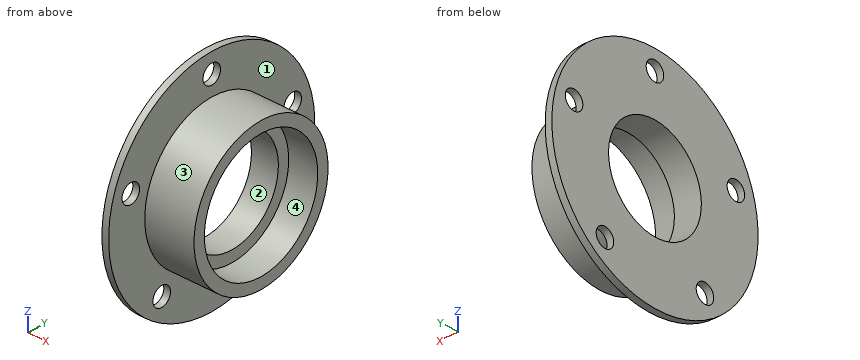
from build123d import *

# Parameters (mm, degrees)
F3_D     = 8.5
F3_DEPTH = 49.5
F3_TIP   = 2.5536576309


# Not quite as in the source:
# - a feature names something its author has since deleted; it is built from what else it names


with BuildPart() as f1:
    # F0 (on Front) → F1 (revolve)
    with BuildSketch(Plane.XZ):
        Polygon((-15.4332816247, 27.5), (-2.4332816247, 27.5), (-2.4332816247, 32.5), (-24.5, 32.5), (-24.5, 50), (-27.5, 50), (-27.5, 22.5), (-15.4332816247, 22.5), align=None)
    revolve(axis=Axis((-62.9697144032, 0, 0), (-1, 0, 0)))

    # F3
    with Locations(Plane(origin=(-27.5, 0, 0), x_dir=(0, -1, 0), z_dir=(-1, 0, 0))):
        with Locations((0, 41.25), (39.2310812972, 12.746951018), (24.2461416571, -33.371951018), (-24.2461416571, -33.371951018), (-39.2310812972, 12.746951018)):
            Hole(F3_D / 2, depth=F3_DEPTH)
            with Locations((0, 0, -(F3_DEPTH + F3_TIP / 2))):  # 118° drill point
                Cone(0, F3_D / 2, F3_TIP, mode=Mode.SUBTRACT)


solid = f1.part
Design review of the part built by this model. Coordinates are the model's own, in mm. Face numbers are marked on the shaded views. Round coordinates to 2 decimals unless told otherwise and drop trailing zeros. Loops run counter-clockwise (first coordinate to the right, second up) from the corner with the lowest first, then second, coordinate; pieces in that order, holes last. Notation, with made-up numbers: M 48,23.25 L 79,23.25 A26 ccw 79,61.25 Z; hole C 13,-25 d4. An arc over 180 degrees is marked long. Answer as a JSON object with one key per item and string values.
Item 1: We need section B-B on z = 11.5. Give the boundary of the cut face in (x, y), and give its area (3 significant figures).
Answer sheet:
{"outline": "M -27.5,-48.66 L -24.5,-48.66 L -24.5,-43.29 L -27.5,-43.29 Z; M -27.5,-35.17 L -24.5,-35.17 L -24.5,-30.4 L -2.43,-30.4 L -2.43,-24.98 L -15.43,-24.98 L -15.43,-19.34 L -27.5,-19.34 Z; M -27.5,19.34 L -15.43,19.34 L -15.43,24.98 L -2.43,24.98 L -2.43,30.4 L -24.5,30.4 L -24.5,35.17 L -27.5,35.17 Z; M -27.5,43.29 L -24.5,43.29 L -24.5,48.66 L -27.5,48.66 Z", "area": "469 mm^2"}
Item 2: We need section C-C on y = -15.5. Give the boundary of the cut face in (x, z).
Answer sheet:
{"outline": "M -27.5,-47.54 L -24.5,-47.54 L -24.5,-28.57 L -2.43,-28.57 L -2.43,-22.72 L -15.43,-22.72 L -15.43,-16.31 L -27.5,-16.31 Z; M -27.5,16.31 L -15.43,16.31 L -15.43,22.72 L -2.43,22.72 L -2.43,28.57 L -24.5,28.57 L -24.5,47.54 L -27.5,47.54 Z"}
Item 3: The part is to be moulded in two halves that separate along Z. For the marked faces 1, 2, 3 and 4, say which applies: pulls with the +Z half, pulls with the -Z half, needs draft (parallel to the pull), parting line crosses it, or undercut.
Answer sheet:
{"face 1": "needs draft", "face 2": "undercut", "face 3": "parting line crosses it", "face 4": "undercut"}
Item 4: We need section D-D on z = 0. Give the boundary of the cut face in (x, y).
Answer sheet:
{"outline": "M -27.5,-50 L -24.5,-50 L -24.5,-32.5 L -2.43,-32.5 L -2.43,-27.5 L -15.43,-27.5 L -15.43,-22.5 L -27.5,-22.5 Z; M -27.5,22.5 L -15.43,22.5 L -15.43,27.5 L -2.43,27.5 L -2.43,32.5 L -24.5,32.5 L -24.5,50 L -27.5,50 Z"}
Item 5: Clearance check with flat-ended pins moving along their axes: P1, Ø1.5, axis at x = -7, y = 29.5, coming from the +Z side; P2, Ø4, axis at x = -10.5, y = -3.5, coming from the -Z side; P3, Ø2, axis at x = -6, z = -6, coming from the -Y side. State where each tip first meets the part, or that it passes through.
Answer sheet:
{"P1": "stops at z = 15.16", "P2": "stops at z = -32.47", "P3": "stops at y = -32.11"}
Item 6: Wall thickness on L1, parallel to Z at x = -21.25, y = -1; L2, parallel to Y at x = -12.75, z = 20; L3, parallel to X at y = -29, z = 26: over which ranges is each line inside the solid? List them lowest first. Write a range as from..to.
Answer sheet:
{"L1": "z = -32.48..-22.48, 22.48..32.48", "L2": "y = -25.62..-18.87, 18.87..25.62", "L3": "x = -27.5..-24.5"}
Item 7: We need section A-A on y = 0. Give the boundary of the cut face in (x, z).
Answer sheet:
{"outline": "M -27.5,-50 L -24.5,-50 L -24.5,-32.5 L -2.43,-32.5 L -2.43,-27.5 L -15.43,-27.5 L -15.43,-22.5 L -27.5,-22.5 Z; M -27.5,22.5 L -15.43,22.5 L -15.43,27.5 L -2.43,27.5 L -2.43,32.5 L -24.5,32.5 L -24.5,37 L -27.5,37 Z; M -27.5,45.5 L -24.5,45.5 L -24.5,50 L -27.5,50 Z"}
